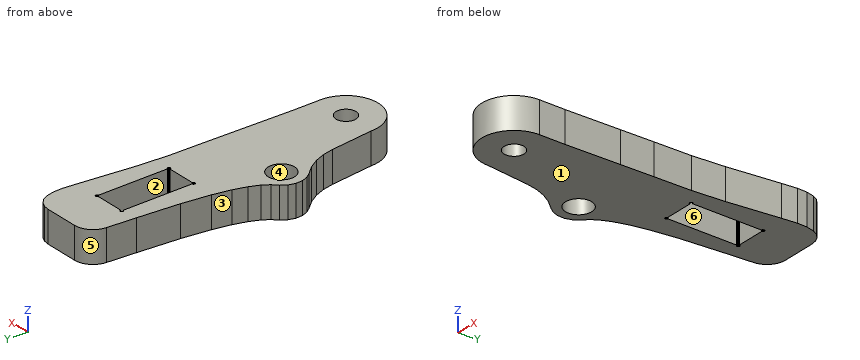
```python
from build123d import *

# Parameters (mm, degrees)
ESQUISSE1_R        = 2.1
ESQUISSE1_R_2      = 1.6
BOSS_EXTRU_1_DEPTH = 5


with BuildPart() as part:
    # Esquisse1 → Boss.-Extru.1 (new body)
    with BuildSketch(Plane.XY.offset(5)):
        with BuildLine():
            Line((21.663586585, 9.246660578), (21.65632273, 5.149368071))
            ThreePointArc((21.65632273, 5.149368071), (16.472816032, -0.006118111), (11.343954037, 5.203733528))
            Line((11.343954037, 5.203733528), (10.574629149, 12.042199031))
            Line((10.574629149, 12.042199031), (10.233579176, 13.737028894))
            Line((10.233579176, 13.737028894), (9.605716227, 15.347798765))
            Line((9.605716227, 15.347798765), (8.709809299, 16.826348646))
            Line((8.709809299, 16.826348646), (7.572636391, 18.128508541))
            Line((7.572636391, 18.128508541), (6.918936443, 18.989558472))
            Line((6.918936443, 18.989558472), (6.559190472, 20.00903839))
            Line((6.559190472, 20.00903839), (6.527723475, 21.089658303))
            Line((6.527723475, 21.089658303), (6.827536451, 22.128338219))
            Line((6.827536451, 22.128338219), (7.430024402, 23.025968147))
            Line((7.430024402, 23.025968147), (8.20419734, 23.752548088))
            Line((8.20419734, 23.752548088), (8.890967284, 24.798538004))
            Line((8.890967284, 24.798538004), (9.556249231, 26.311877882))
            Line((9.556249231, 26.311877882), (10.18684918, 28.409207714))
            Line((10.18684918, 28.409207714), (10.765999134, 31.224477487))
            Line((10.765999134, 31.224477487), (11.369489085, 35.732217124))
            Line((11.369489085, 35.732217124), (11.92756904, 42.336066593))
            Line((11.92756904, 42.336066593), (12.268069386, 46.901117167))
            ThreePointArc((12.268069386, 46.901117167), (13.209278732, 48.85686853), (15.229621264, 49.649998078))
            Line((15.229621264, 49.649998078), (20.556119459, 49.649998078))
            Line((20.556119459, 49.649998078), (21.457249103, 49.511456244))
            Line((21.457249103, 49.511456244), (22.275158213, 49.108634602))
            Line((22.275158213, 49.108634602), (22.93428687, 48.478733303))
            Line((22.93428687, 48.478733303), (23.373775199, 47.679942467))
            Line((23.373775199, 47.679942467), (23.668052623, 46.433641965))
            Line((23.668052623, 46.433641965), (23.713799348, 44.835742))
            Line((23.713799348, 44.835742), (23.469414511, 42.463982691))
            Line((23.469414511, 42.463982691), (22.514057727, 34.22916531))
            Line((22.514057727, 34.22916531), (22.119847298, 29.119826528))
            Line((22.119847298, 29.119826528), (22.000035211, 23.212167249))
            Line((22.000035211, 23.212167249), (21.870164382, 17.918027941))
            Line((21.870164382, 17.918027941), (21.663586585, 9.246660578))
        make_face()
        with Locations((9.999996695, 20.649998987)):
            Circle(ESQUISSE1_R, mode=Mode.SUBTRACT)
        with Locations((16.499999118, 5.150133907)):
            Circle(ESQUISSE1_R_2, mode=Mode.SUBTRACT)
        Polygon((14.249998853, 42.649996567), (14.28348885, 42.774996557), (14.374998843, 42.86649655), (14.499998833, 42.899996547), (14.624998823, 42.86649655), (14.716508816, 42.774996557), (14.749998813, 42.649996567), (19.249998451, 42.649996567), (19.283488448, 42.774996557), (19.374998441, 42.86649655), (19.499998431, 42.899996547), (19.624998421, 42.86649655), (19.716508413, 42.774996557), (19.74999841, 42.649996567), (19.716508413, 42.524996577), (19.624998421, 42.433486585), (19.499998431, 42.399996588), (19.499998431, 31.399997473), (19.624998421, 31.366497476), (19.716508413, 31.274997483), (19.74999841, 31.149997493), (19.716508413, 31.024997503), (19.624998421, 30.93348751), (19.499998431, 30.899997513), (19.374998441, 30.93348751), (19.283488448, 31.024997503), (19.249998451, 31.149997493), (14.749998813, 31.149997493), (14.716508816, 31.024997503), (14.624998823, 30.93348751), (14.499998833, 30.899997513), (14.374998843, 30.93348751), (14.28348885, 31.024997503), (14.249998853, 31.149997493), (14.28348885, 31.274997483), (14.374998843, 31.366497476), (14.499998833, 31.399997473), (14.499998833, 42.399996588), (14.374998843, 42.433486585), (14.28348885, 42.524996577), align=None, mode=Mode.SUBTRACT)
    extrude(amount=-BOSS_EXTRU_1_DEPTH)


solid = part.part
```
Verification items for the finished model (mm, model axes). Face numbers are marked on the shaded views. A direction names the side the tool comes from. Coordinates: 2 decimals unless noted, no trailing zeros. Order: outer loops, then holes, each group sorted by start corner. A loop starts at its lowest first (then second) coordinate and runs counter-clockwise, first axis right, second up. Notation, with made-up numbers: (-17, 76) -> (18, 76) arc R11 cw to (18, 96) -> close; hole circle Ø4 at (70, 12). An arc over 180 degrees is marked (long way). Put each result on its own line as item: value. Start each with the question number.
1) Cross-section at C-C (z = 0.6). State how many separate pieces and enclosed holes the cut face has, plus the area to 3 significant figures.
2) Cross-section at B-B (y = 39.5). Enter the section's corners in (x, z).
3) Go/stop test with flat-tipped pins: pin 1 (1.5 mm diameter, centred on y = 28.5, z = 3.5, fed in from +X); pin 2 (1 mm diameter, centred on y = 41, z = 1.5, fed in from -X); pin 3 (2.5 mm diameter, centred on y = 38.5, z = 1.5, fed in from +X); pin 4 (4 mm diameter, centred on x = 22, y = 19, fed in from -Z). Record where each tip stops, or that it passes through.
4) Tool access check on the marked faces 5 and 6. Record the directions out of +Z, -Z, +X, -X, +Y, -Y that give a thin tool (end or side, any length) a straight path to the whole face; none if there is none.
5) Release check for a two-part mould opening along Y. For the marked faces 1, 2, 3 and 4 record: pulls with the +Y half, pulls with the -Y half, needs draft (parallel to the pull), parting line crosses it, or undercut.
6) Cross-section at D-D (x = 21). Enter the section's corners in (y, z).
7) Material ranges on L1, parallel to Y at x = 16.5, z = 3.05; L2, parallel to Y at x = 17.75, z = 2.5; L3, parallel to X at y = 42, z = 3.5, recorded low to high.
8) Cross-section at A-A (x = 16.5). Enter the section's corners in (y, z), plus the area to 3 significant figures.
Geometry check:
1. separate pieces: 1
1. enclosed holes: 3
1. area: 493 mm^2
2. outline: (11.69, 0) -> (14.5, 0) -> (14.5, 5) -> (11.69, 5) -> close; (19.5, 0) -> (23.13, 0) -> (23.13, 5) -> (19.5, 5) -> close
3. pin 1: stops at x = 22.13
3. pin 2: stops at x = 11.77
3. pin 3: stops at x = 23.15
3. pin 4: stops at z = 0
4. face 5: +Z, -Z, -X, +Y
4. face 6: +Z, -Z
5. face 1: needs draft
5. face 2: undercut
5. face 3: pulls with the +Y half
5. face 4: undercut
6. outline: (2.63, 0) -> (49.58, 0) -> (49.58, 5) -> (2.63, 5) -> close
7. L1: y = -0.01 to 3.55, 6.75 to 31.15, 42.65 to 49.65
7. L2: y = 0.15 to 4.15, 6.15 to 31.15, 42.65 to 49.65
7. L3: x = 11.9 to 14.5, 19.5 to 23.42
8. outline: (-0.01, 0) -> (3.55, 0) -> (3.55, 5) -> (-0.01, 5) -> close; (6.75, 0) -> (31.15, 0) -> (31.15, 5) -> (6.75, 5) -> close; (42.65, 0) -> (49.65, 0) -> (49.65, 5) -> (42.65, 5) -> close
8. area: 175 mm^2
